```python
from build123d import *

# Parameters (mm, degrees)
SKETCH_R      = 4
SKETCH_R_2    = 2.5
SKETCH_R_3    = 1.5
PAD_DEPTH     = 4
SKETCH001_R   = 9
SKETCH001_R_2 = 4
PAD001_DEPTH  = 8
SKETCH002_R   = 4
PAD002_DEPTH  = 3
PAD003_DEPTH  = 1.5
SKETCH004_R   = 5
SKETCH004_R_2 = 2.5
PAD004_DEPTH  = 2
CHAMFER_SIZE  = 0.6
SKETCH005_R   = 1.35
PAD005_DEPTH  = 2


with BuildPart() as part:
    # Sketch → Pad (new body)
    with BuildSketch(Plane.XY):
        with BuildLine():
            ThreePointArc((7.483315, 5), (-9, 0), (7.483315, -5))
            Line((7.483315, -5), (100.516685, -5))
            ThreePointArc((100.516685, -5), (117, 0), (100.516685, 5))
            Line((7.483315, 5), (100.516685, 5))
        make_face()
        Circle(SKETCH_R, mode=Mode.SUBTRACT)
        with Locations((108, 0)):
            Circle(SKETCH_R, mode=Mode.SUBTRACT)
        with Locations((39, 0)):
            Circle(SKETCH_R_2, mode=Mode.SUBTRACT)
        with Locations((79, 0)):
            Circle(SKETCH_R_2, mode=Mode.SUBTRACT)
        with Locations((72.5, 0)):
            Circle(SKETCH_R_3, mode=Mode.SUBTRACT)
        with Locations((68.5, 0)):
            Circle(SKETCH_R_3, mode=Mode.SUBTRACT)
    extrude(amount=PAD_DEPTH)

    # Sketch001 (on Face12 of Pad) → Pad001 (join)
    with BuildSketch(Plane.XY.offset(4)):
        Circle(SKETCH001_R)
        Circle(SKETCH001_R_2, mode=Mode.SUBTRACT)
        with Locations((108, 0)):
            Circle(SKETCH001_R)
        with Locations((108, 0)):
            Circle(SKETCH001_R_2, mode=Mode.SUBTRACT)
    extrude(amount=PAD001_DEPTH)

    # Sketch002 (on Face4 of Pad001) → Pad002 (join)
    with BuildSketch(Plane(origin=(0, 0, 0), x_dir=(1, 0, 0), z_dir=(0, 0, -1))):
        with Locations((108, 0)):
            Circle(SKETCH002_R)
        Circle(SKETCH002_R)
    extrude(amount=-PAD002_DEPTH)

    # Sketch003 (on Face3 of Pad002) → Pad003 (join, symmetric)
    with BuildSketch(Plane.XZ):
        Polygon((100, 12), (100, 4), (83.5, 4), (83.5, 6), (89.5, 12), align=None)
        Polygon((8, 4), (8, 12), (28.5, 12), (34.5, 6), (34.5, 4), align=None)
        Polygon((43.5, 4), (67, 4), (67, 6), (61, 12), (49.5, 12), (43.5, 6), align=None)
    extrude(amount=PAD003_DEPTH, both=True)

    # Sketch004 (on Face7 of Pad003) → Pad004 (join)
    with BuildSketch(Plane.XY.offset(4)):
        with Locations((39, 0)):
            Circle(SKETCH004_R)
        with Locations((39, 0)):
            Circle(SKETCH004_R_2, mode=Mode.SUBTRACT)
        with Locations((79, 0)):
            Circle(SKETCH004_R)
        with Locations((79, 0)):
            Circle(SKETCH004_R_2, mode=Mode.SUBTRACT)
    extrude(amount=PAD004_DEPTH)

    # Chamfer
    chamfer_edges = [part.edges().sort_by_distance(p)[0] for p in [
        (-4, 0, 12),
        (104, 0, 12),
    ]]
    chamfer(chamfer_edges, length=CHAMFER_SIZE)

    # Sketch005 (on Face22 of Chamfer) → Pad005 (join)
    with BuildSketch(Plane.XY.offset(4)):
        with BuildLine():
            ThreePointArc((70.5, 4.582576), (63.5, 0), (70.5, -4.582576))
            ThreePointArc((70.5, -4.582576), (73.237469, -4.945315), (75.75, -3.799671))
            ThreePointArc((75.75, 3.799671), (74, 0), (75.75, -3.799671))
            ThreePointArc((75.75, 3.799671), (73.237469, 4.945315), (70.5, 4.582576))
        make_face()
        with Locations((68.5, 0)):
            Circle(SKETCH005_R, mode=Mode.SUBTRACT)
        with Locations((72.5, 0)):
            Circle(SKETCH005_R, mode=Mode.SUBTRACT)
    extrude(amount=PAD005_DEPTH)


solid = part.part
```
The listing builds one solid part. Answer for the finished solid, in the listing's coordinates (mm). A direction names the side the tool comes from. Give positions to 0.01 mm unless a question says otherwise; leave off trailing zeros. Write each loop counter-clockwise with the first axis right and the second up, starting at its lowest first coordinate (ties: lowest second). Pieces come first, ordered by that corner, then holes. Notation, with made-up numbers: (58, 25.5) - (105, 25.5) arc R10 ccw to (105, 38.5) - close; hole circle Ø8 at (30, 11.5). An arc over 180 degrees is marked (long way). Use one line per item in the form item = value. Start each with the question number.
1) Find section D-D on x = 108. Determine the outline of the cut face in (y, z), plus the area to 3 significant figures.
2) Find section C-C on y = 7. Determine the outline of the cut face in (x, z).
3) Find section A-A on z = 10.25. Determine the outline of the cut face in (x, y).
4) Consider line 1 along Y through (x, z) = (68.5, 3.1); line 2 along X through (y, z) = (0, 8.75); line 3 along X through (y, z) = (2, 2.5). Determine where each line is inside the solid, lowest interval first. Write a range as from..to.
5) Find section B-B on x = 14. Determine the outline of the cut face in (y, z).
6) Flat-ended cylindrical pins translate along their axes: pin 1 Ø6 at (x, y) = (28, 6) entering from +Z; pin 2 Ø3 at (x, y) = (75.5, 5.5) entering from -Z; pin 3 Ø8 at (x, y) = (79, 0) entering from +Z; pin 4 Ø4 at (x, y) = (1.5, 1) entering from +Z. Find the tip coordinate at first contact, or state that the pin passes through.
7) A tool of negligible diameter and unlimited length cuts with its end or side. For faces 1 (the face through (80.4, 4.8, 5)), 2 (the face through (31.5, 0, 9)), 3 (the face through (39, -5, 5)), 4 (the face through (70, 0, 2)), from which of +Z, -Z, +X, -X, +Y, -Y can it reach the whole face along a straight path? Write none if from no direction.
Geometry results:
q1.outline = (-9, 0) - (9, 0) - (9, 12) - (4.6, 12) - (4, 11.4) - (4, 3) - (-4, 3) - (-4, 11.4) - (-4.6, 12) - (-9, 12) - close
q1.area = 144 mm2
q2.outline = (-5.66, 0) - (5.66, 0) - (5.66, 12) - (-5.66, 12) - close; (102.34, 0) - (113.66, 0) - (113.66, 12) - (102.34, 12) - close
q3.outline = (8.87, -1.5) - (30.25, -1.5) - (30.25, 1.5) - (8.87, 1.5) arc R9 ccw (long way) to start; (47.75, -1.5) - (62.75, -1.5) - (62.75, 1.5) - (47.75, 1.5) - close; (87.75, -1.5) - (99.13, -1.5) arc R9 ccw (long way) to (99.13, 1.5) - (87.75, 1.5) - close; hole circle Ø8 at (0, 0); hole circle Ø8 at (108, 0)
q4.line_1 = -5..-1.5, 1.5..5
q4.line_2 = -9..-4, 4..31.75, 46.25..64.25, 86.25..104, 112..117
q4.line_3 = -8.77..37.5, 40.5..77.5, 80.5..116.77
q5.outline = (-5, 0) - (5, 0) - (5, 4) - (1.5, 4) - (1.5, 12) - (-1.5, 12) - (-1.5, 4) - (-5, 4) - close
q6.pin_1 = 4
q6.pin_2 = 0
q6.pin_3 = 6
q6.pin_4 = 3
q7.face_1 = +Z, +Y
q7.face_2 = +Z, +Y, -Y
q7.face_3 = +Z, -Y
q7.face_4 = -Z
